Can you work these out from the drawing? Everything is in mm from the part's minimum corner. A direction names the side the tool comes from. Give positions to 0.01 mm unless a question says otherwise; leave off trailing zeros. Write each loop counter-clockwise with the first axis right and the second up, starting at its lowest first coordinate (ties: lowest second). Pieces come first, ordered by that corner, then holes. Notation, with made-up numbers: (53, -14) - (84, -14) arc R12 cw to (84, -8) - close; hole circle Ø4 at (56.25, -12). An arc over 180 degrees is marked (long way). Use a Markdown table: item, result.
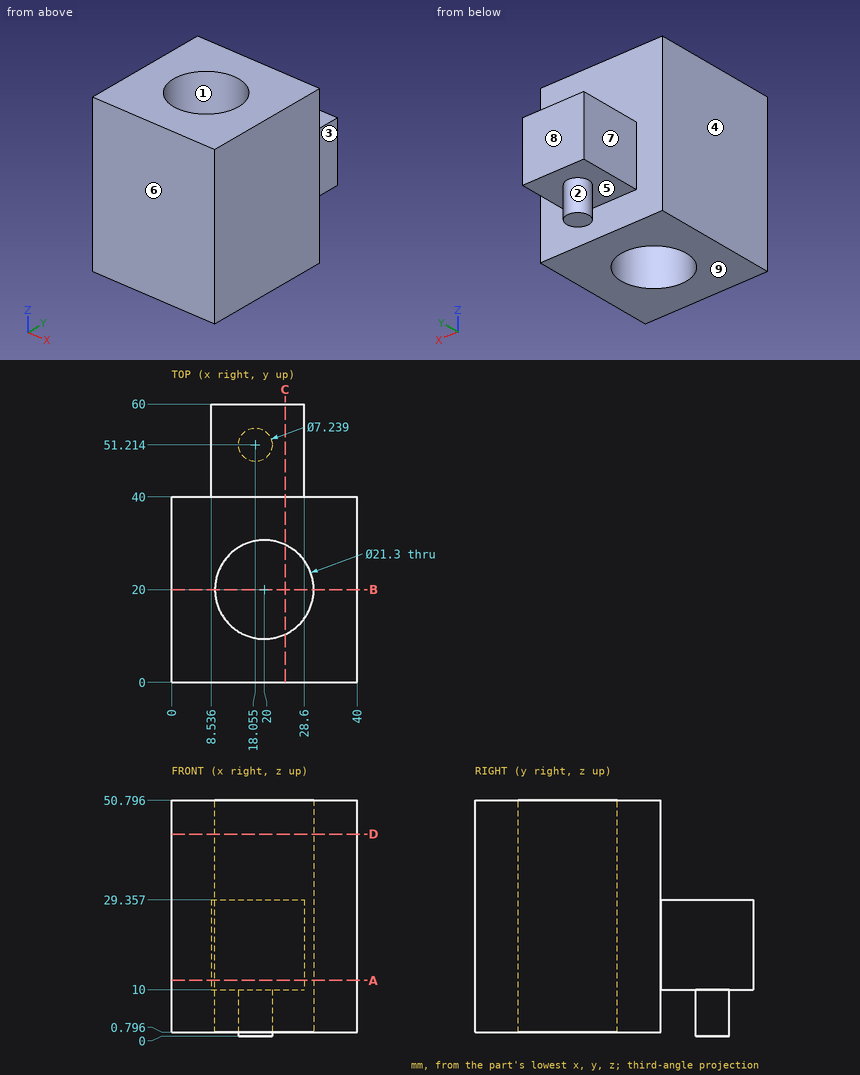
Item 1: If we section it at C-C, the plane x = 24.5: Write out the boundary of the cut face in (y, z).
Values:
| item | result |
|---|---|
| outline | (0, 0.8) - (10.35, 0.8) - (10.35, 50.8) - (0, 50.8) - close; (29.65, 0.8) - (40, 0.8) - (40, 10) - (60, 10) - (60, 29.36) - (40, 29.36) - (40, 50.8) - (29.65, 50.8) - close |
Item 2: I need wall thicknesses on line 1 along Y through (x, z) = (20, 29); line 2 along X through (y, z) = (19.5, 31); line 3 along Z through (x, y) = (31.5, 31.5). Which ranges of each line are inside material? Lowest first, please. Write a range as [from, to].
Values:
| item | result |
|---|---|
| line 1 | y = [0, 9.35], [30.65, 60] |
| line 2 | x = [0, 9.36], [30.64, 40] |
| line 3 | z = [0.8, 50.8] |
Item 3: Will these pins go through, and if not, where does the flat tip stop? pin 1 Ø21.5 at (y, z) = (48.5, 23) entering from -X; pin 2 Ø2 at (x, z) = (15, 6) entering from +Y; pin 3 Ø6 at (y, z) = (50, 20.5) entering from +X; pin 4 Ø3 at (x, z) = (27.5, 35.5) entering from +Y.
Values:
| item | result |
|---|---|
| pin 1 | stops at x = 0 |
| pin 2 | stops at y = 54.19 |
| pin 3 | stops at x = 28.6 |
| pin 4 | stops at y = 40 |
Item 4: For the marked faces 5, 6, 7, 8 and 9, which set-ups out of +Z, -Z, +X, -X, +Y, -Y let a thin tool reach every point of the face, with its end or its side?
Values:
| item | result |
|---|---|
| face 5 | -Z |
| face 6 | +Z, -Z, +X, -X, -Y |
| face 7 | +Z, -Z, -X, +Y |
| face 8 | +Z, -Z, +X, -X, +Y |
| face 9 | -Z, +X, -X, -Y |
Item 5: Thinking about a two-plate mould opening in X: for the marked faces 1, 2, 3 and 4, which applies, +X half, -X half, draft (parallel to the pull), parting line (faces both ways), or undercut?
Values:
| item | result |
|---|---|
| face 1 | undercut |
| face 2 | parting line |
| face 3 | +X half |
| face 4 | -X half |
Item 6: If we section it at A-A, the plane z = 12: Write out the boundary of the cut face in (x, y), plus the area to 4 significant figures.
Values:
| item | result |
|---|---|
| outline | (0, 0) - (40, 0) - (40, 40) - (28.6, 40) - (28.6, 60) - (8.54, 60) - (8.54, 40) - (0, 40) - close; hole circle Ø21.3 at (20, 20) |
| area | 1,645 mm2 |
Item 7: If we section it at D-D, the plane z = 43.5: Write out the boundary of the cut face in (x, y), plus the area to 3 significant figures.
Values:
| item | result |
|---|---|
| outline | (0, 0) - (40, 0) - (40, 40) - (0, 40) - close; hole circle Ø21.3 at (20, 20) |
| area | 1,240 mm2 |
Item 8: If we section it at B-B, the plane y = 20: Write out the boundary of the cut face in (x, z), plus the area to 3 significant figures.
Values:
| item | result |
|---|---|
| outline | (0, 0.8) - (9.35, 0.8) - (9.35, 50.8) - (0, 50.8) - close; (30.65, 0.8) - (40, 0.8) - (40, 50.8) - (30.65, 50.8) - close |
| area | 935 mm2 |
